For this review, take the finished solid that the model builds, in its own axes (mm). A direction names the side the tool comes from. Give positions to 0.01 mm unless a question says otherwise; leave off trailing zeros. Loops run counter-clockwise (first coordinate to the right, second up) from the corner with the lowest first, then second, coordinate; pieces in that order, holes last. Notation, with made-up numbers: (23.25, 32.25) - (29.25, 32.25) arc R7 cw to (29.25, 41.25) - close; hole circle Ø10 at (70.5, 21.5). An arc over 180 degrees is marked (long way). Answer as CSV lines item,"result".
Autodesk Inventor part; units mm, degrees
ref_plane "YZ Plane" through (0, 0, 0) normal (1, 0, 0) x (0, 1, 0)
ref_plane "XZ Plane" through (0, 0, 0) normal (0, 1, 0) x (-1, 0, 0)
ref_plane "XY Plane" through (0, 0, 0) normal (0, 0, 1) x (1, 0, 0)
sketch "Sketch1" plane through (0, 0, 0) normal (0, 0, 1) x (1, 0, 0)
  line L0 (-37.5, 19) -> (37.5, 19)
  line L1 (37.5, 19) -> (37.5, -19)
  line L2 (37.5, -19) -> (-37.5, -19)
  line L3 (-37.5, -19) -> (-37.5, 19)
  line L4 (-37.5, 19) -> (37.5, -19) construction
  line L5 (37.5, 19) -> (-37.5, -19) construction
  point P0 (0, 0)
  dimension "d2" = 38
  dimension "d3" = 75
extrude "Extrusion1" add sketch "Sketch1" along normal mid plane 10
sketch "Sketch3" plane through (0, 0, 5) normal (0, 0, 1) x (1, 0, 0)
  point P0 (0, 0)
  point P1 (0, 0)
hole "Hole2" at (0, 0, 5) direction (0, 0, -1) diameter 3.175 depth 5 tip angle 118
sketch "Sketch4" plane through (0, 0, 5) normal (0, 0, 1) x (1, 0, 0)
  line L0 (-37.5, 19) -> (-37.5, -19)
  circle A0 centre (0, 0) radius 1.5875
  line L1 (-37.5, -19) -> (37.5, -19)
  line L2 (37.5, -19) -> (37.5, 19)
  line L3 (37.5, 19) -> (-37.5, 19)
  line L4 (-37.5, 19) -> (-37.5, -19)
  point P0 (-32.5, 0)
  point P1 (32.5, 0)
  dimension "d76" = 5
  dimension "d79" = 65
hole "Hole3" at (-32.5, 0, 5) at (32.5, 0, 5) direction (0, 0, -1) diameter 3.242 end through all
properties part number "baseblock"
1) Machinability: for faces 1 (the cylindrical face through (34.082, 0.351, -0.07)), 2 (the cylindrical face through (1.55, 0.34, 2.46)), which of the approach directions +Z, -Z, +X, -X, +Y, -Y give a long, thin tool a straight path to every point of the face, cutting with its end or side? Answer none if there is none.
From the geometry:
face 1,"+Z, -Z"
face 2,"+Z"
2) Insertion check: P1, Ø3, axis at x = -32.5, y = 0, coming from the +Z side. The pin has a flat end and moves straight along its axis. Give the tip position at first contact, or say it passes through.
From the geometry:
P1,"passes through"
3) Consider section A-A on x = -32.5. Write out the cut boundary in (y, z).
From the geometry:
outline,"(-19, -5) - (-1.62, -5) - (-1.62, 5) - (-19, 5) - close; (1.62, -5) - (19, -5) - (19, 5) - (1.62, 5) - close"
4) Wall thickness on line 1 (X direction, y = 0, z = -1.5); line 2 (X direction, y = 0, z = 1.5); line 3 (Y direction, x = 32.5, z = -0.25): over which ranges is each line inside the solid? List them lowest first. Write a range as from..to.
From the geometry:
line 1,"x = -37.5..-34.12, -30.88..30.88, 34.12..37.5"
line 2,"x = -37.5..-34.12, -30.88..-1.59, 1.59..30.88, 34.12..37.5"
line 3,"y = -19..-1.62, 1.62..19"
